Could you check a few things on this model? Use its own coordinates, in mm. A direction names the side the tool comes from. Coordinates: 2 decimals unless noted, no trailing zeros. Loops run counter-clockwise (first coordinate to the right, second up) from the corner with the lowest first, then second, coordinate; pieces in that order, holes last.
from build123d import *

# Parameters (mm, degrees)
F1_DEPTH    = 30
F2_R        = 5
F3_T1_DEPTH = 54.4948974279
F3_T3_DEPTH = 55
F4_R        = 5
F6_D        = 6


# Not quite as in the source:
# - a fillet or chamfer that OpenCascade refuses, or shapes differently, is made with other operations: its cross-section is extruded or revolved along the edge and cut away or added


with BuildPart() as f1:
    # F0 (on Front) → F1 (new body)
    with BuildSketch(Plane.XZ):
        with BuildLine():
            Line((0, 30), (0, 0))
            Line((0, 0), (9.5, 0))
            Line((9.5, 0), (9.5, 6))
            ThreePointArc((9.5, 6), (10.2639320225, 14.472135955), (17.5, 10))
            ThreePointArc((17.5, 10), (16.972135955, 7.7639320225), (15.5, 6))
            Line((15.5, 6), (15.5, 0))
            Line((15.5, 0), (34.5, 0))
            Line((34.5, 0), (34.5, 6))
            ThreePointArc((34.5, 6), (35.2639320225, 14.472135955), (42.5, 10))
            ThreePointArc((42.5, 10), (41.972135955, 7.7639320225), (40.5, 6))
            Line((40.5, 6), (40.5, 0))
            Line((40.5, 0), (50, 0))
            Line((50, 0), (50, 30))
            Line((50, 30), (0, 30))
        make_face()
    extrude(amount=F1_DEPTH)

    # F2
    f2_edges = [f1.edges().sort_by_distance(p)[0] for p in [
        (40.5, -15, 6),
        (34.5, -15, 6),
        (9.5, -15, 6),
        (15.5, -15, 6),
    ]]
    fillet(f2_edges, radius=F2_R)

    # F3: fillet of radius 5 on 6 edges, made by hand

    # F3_s2 → F3_t1 (cut)
    with BuildSketch(Plane.XZ.offset(-12.2474487139)):
        with BuildLine():
            ThreePointArc((4.6010205144, 0), (7.7632981746, 1.1270166538), (9.5, 4))
            Line((9.5, 4), (9.5, 0))
            Line((9.5, 0), (4.6010205144, 0))
        make_face()
        with BuildLine():
            ThreePointArc((34.5, 4), (32.7632981746, 1.1270166538), (29.6010205144, 0))
            Line((29.6010205144, 0), (34.5, 0))
            Line((34.5, 0), (34.5, 4))
        make_face()
        with BuildLine():
            ThreePointArc((40.5, 4), (42.2367018254, 1.1270166538), (45.3989794856, 0))
            Line((45.3989794856, 0), (40.5, 0))
            Line((40.5, 0), (40.5, 4))
        make_face()
        with BuildLine():
            ThreePointArc((20.3989794856, 0), (17.2367018254, 1.1270166538), (15.5, 4))
            Line((15.5, 4), (15.5, 0))
            Line((15.5, 0), (20.3989794856, 0))
        make_face()
    extrude(amount=F3_T1_DEPTH, mode=Mode.SUBTRACT)

    # F3_s4 → F3_t3 (cut)
    with BuildSketch(Plane.XZ.offset(-12.5)):
        with BuildLine():
            ThreePointArc((45, 0), (48.5355339059, 1.4644660941), (50, 5))
            Line((50, 5), (50, 0))
            Line((50, 0), (45, 0))
        make_face()
        with BuildLine():
            ThreePointArc((0, 5), (1.4644660941, 1.4644660941), (5, 0))
            Line((5, 0), (0, 0))
            Line((0, 0), (0, 5))
        make_face()
    extrude(amount=F3_T3_DEPTH, mode=Mode.SUBTRACT)

    # F4
    f4_edges = [f1.edges().sort_by_distance(p)[0] for p in [
        (25, -30, 30),
        (25, 0, 30),
    ]]
    fillet(f4_edges, radius=F4_R)

    # F6 (through all)
    with Locations(Plane.YZ.offset(50)):
        with Locations((-15, 22)):
            Hole(F6_D / 2)


solid = f1.part
1) If I drill on L1, parallel to X at y = -28, z = 10; L2, parallel to Z at x = 28.5, y = -15; L3, parallel to X at y = -11, z = 2, over which ranges is the centre line in solid material (lowest first)?
2) For faces 5 (the flat face through (0, -15, 18)), 6 (the cylindrical face through (17.27, -14.79, 1.1)), which set-ups out of +Z, -Z, +X, -X, +Y, -Y let a thin tool reach every point of the face, with its end or its side?
3) Imagine slicing it at A-A on z = 22. List the corners of the cut face in (x, y) for me.
4) Will these pins go through, and if not, where does the flat tip stop? pin 1 (6 mm diameter, centred on x = 39.5, z = 6.5, fed in from +Y); pin 2 (6 mm diameter, centred on x = 12.5, z = 10, fed in from +Y); pin 3 (1.5 mm diameter, centred on x = 39, y = -11, fed in from -Z).
5) We'd pull the mould along Z, two halves only. Please class faces 1 (the cylindrical face through (25, -1, 28)), 2 (the flat face through (25, 0, 13)), 3 (the cylindrical face through (24.7, -12.6, 20.2)), 4 (the cylindrical face through (42.125, -14.79, 1.221)): released by +Z, released by -Z, zero draft, split by the parting line, or undercut.
6) Imagine slicing it at D-D on x = 12.5. List the corners of the cut face in (y, z) for me, plus the area to 3 significant figures.
7) Imagine slicing it at C-C on z = 10. List the corners of the cut face in (x, y) for me, plus the area to 3 significant figures.
8) Imagine slicing it at B-B on y = -15. List the corners of the cut face in (x, z) for me, plus the area to 3 significant figures.
Solved:
1. L1: x = 0 to 7.5, 17.5 to 32.5, 42.5 to 50
1. L2: z = 0 to 19, 25 to 30
1. L3: x = 1 to 8.6, 16.4 to 33.6, 41.4 to 49
2. face 5: +Z, -Z, -X, +Y, -Y
2. face 6: -Z, +Y, -Y
3. outline: (0, -30) - (50, -30) - (50, -18) - (0, -18) - close; (0, -12) - (50, -12) - (50, 0) - (0, 0) - close
4. pin 1: stops at y = 0
4. pin 2: passes through
4. pin 3: stops at z = 14.47
5. face 1: released by +Z
5. face 2: zero draft
5. face 3: undercut
5. face 4: released by -Z
6. outline: (-30, 15) - (0, 15) - (0, 25) arc R5 ccw to (-5, 30) - (-25, 30) arc R5 ccw to (-30, 25) - close; hole circle Ø6 at (-15, 22)
6. area: 411 mm2
7. outline: (0, -30) - (7.5, -30) - (7.5, 0) - (0, 0) - close; (17.5, -30) - (32.5, -30) - (32.5, 0) - (17.5, 0) - close; (42.5, -30) - (50, -30) - (50, 0) - (42.5, 0) - close
7. area: 900 mm2
8. outline: (0, 5) arc R5 ccw to (4.8, 0) arc R5 ccw to (9.5, 4) arc R5 ccw to (8.5, 7) arc R5 cw (long way) to (16.5, 7) arc R5 ccw to (15.5, 4) arc R5 ccw to (20.4, 0) - (29.6, 0) arc R5 ccw to (34.5, 4) arc R5 ccw to (33.5, 7) arc R5 cw (long way) to (41.5, 7) arc R5 ccw to (40.5, 4) arc R5 ccw to (45.2, 0) arc R5 ccw to (50, 5) - (50, 19) - (0, 19) - close; (0, 25) - (50, 25) - (50, 30) - (0, 30) - close
8. area: 947 mm2
